Geometry: final body of the model. Coordinates: model frame, mm. A direction names the side the tool comes from. Give positions to 0.01 mm unless a question says otherwise; leave off trailing zeros. Order: outer loops, then holes, each group sorted by start corner. A loop starts at its lowest first (then second) coordinate and runs counter-clockwise, first axis right, second up. Notation, with made-up numbers: (87, 37) - (94, 37) arc R28 ccw to (94, 73) - close; hole circle Ø4 at (28.5, 21.5). An arc over 180 degrees is marked (long way). Use one line per item in the form item = value.
from build123d import *

# Parameters (mm, degrees)
SKETCH1_R             = 14.29385
SKETCH1_R_2           = 11.1125
BOSS_EXTRUDE1_DEPTH   = 6.35
CROQUIS1_R            = 2.38125
CORTAR_EXTRUIR1_DEPTH = 50
CROQUIS4_R            = 5
CORTAR_EXTRUIR2_DEPTH = 3.175
CROQUIS5_R            = 5
CORTAR_EXTRUIR3_DEPTH = 3.175
CROQUIS6_R            = 2.38125
CORTAR_EXTRUIR4_DEPTH = 10
CROQUIS7_R            = 2.38125
CORTAR_EXTRUIR5_DEPTH = 10
CROQUIS8_R            = 5
CORTAR_EXTRUIR6_DEPTH = 3.16


with BuildPart() as part:
    # Sketch1 → Boss-Extrude1 (new body)
    with BuildSketch(Plane.XY):
        with BuildLine():
            Line((0, 70), (310, 45))
            ThreePointArc((310, 45), (355, 0), (310, -45))
            Line((310, -45), (5.171398252, -69.808714643))
            ThreePointArc((5.171398252, -69.808714643), (-69.952162315, -2.587467389), (0, 70))
        make_face()
        Circle(SKETCH1_R, mode=Mode.SUBTRACT)
        with Locations((310, 0)):
            Circle(SKETCH1_R, mode=Mode.SUBTRACT)
        with Locations((162.878542763, 35)):
            Circle(SKETCH1_R_2, mode=Mode.SUBTRACT)
        with BuildLine():
            Line((107.898974887, 49.259511156), (143.314248041, 46.40344074))
            ThreePointArc((143.314248041, 46.40344074), (147.389908855, 43.644764005), (147.127454118, 38.730252238))
            Line((147.127454118, 38.730252238), (129.916226305, 11.754586611))
            ThreePointArc((129.916226305, 11.754586611), (125.651076231, 9.444205574), (121.433006579, 11.839462159))
            Line((121.433006579, 11.839462159), (103.228961238, 41.671198203))
            ThreePointArc((103.228961238, 41.671198203), (103.238833139, 46.896293531), (107.898974887, 49.259511156))
        make_face(mode=Mode.SUBTRACT)
        with BuildLine():
            Line((70.523244027, 6), (102.03004784, 6))
            ThreePointArc((102.03004784, 6), (106.3902351, 8.552804247), (106.298140539, 13.604493178))
            Line((106.298140539, 13.604493178), (96.590354482, 29.513051181))
            ThreePointArc((96.590354482, 29.513051181), (88.437172177, 34.296727565), (79.941746192, 30.151166228))
            Line((79.941746192, 30.151166228), (65.58297828, 10.229432452))
            ThreePointArc((65.58297828, 10.229432452), (67.271539685, 7.201787411), (70.523244027, 6))
        make_face(mode=Mode.SUBTRACT)
        with BuildLine():
            Line((219.623774494, 32.810522613), (206.130928429, 12.417497436))
            ThreePointArc((206.130928429, 12.417497436), (201.919524559, 10.176643248), (197.745901529, 12.48710226))
            Line((197.745901529, 12.48710226), (183.296864227, 35.133505128))
            ThreePointArc((183.296864227, 35.133505128), (183.227765467, 40.400743015), (187.913912204, 42.80669363))
            Line((187.913912204, 42.80669363), (215.855795571, 40.553315939))
            ThreePointArc((215.855795571, 40.553315939), (219.949772588, 37.757395035), (219.623774494, 32.810522613))
        make_face(mode=Mode.SUBTRACT)
        with BuildLine():
            Line((96.590354482, -29.513051181), (106.298140539, -13.604493178))
            ThreePointArc((106.298140539, -13.604493178), (106.3902351, -8.552804247), (102.03004784, -6))
            Line((102.03004784, -6), (70.523244027, -6))
            ThreePointArc((70.523244027, -6), (67.271539685, -7.201787411), (65.58297828, -10.229432452))
            Line((65.58297828, -10.229432452), (79.941746192, -30.151166228))
            ThreePointArc((79.941746192, -30.151166228), (88.437172177, -34.296727565), (96.590354482, -29.513051181))
        make_face(mode=Mode.SUBTRACT)
        with BuildLine():
            Line((187.913912204, -42.80669363), (215.855795571, -40.553315939))
            ThreePointArc((215.855795571, -40.553315939), (219.949772588, -37.757395035), (219.623774494, -32.810522613))
            Line((219.623774494, -32.810522613), (206.130928429, -12.417497436))
            ThreePointArc((206.130928429, -12.417497436), (201.919524559, -10.176643248), (197.745901529, -12.48710226))
            Line((197.745901529, -12.48710226), (183.296864227, -35.133505128))
            ThreePointArc((183.296864227, -35.133505128), (183.227765467, -40.400743015), (187.913912204, -42.80669363))
        make_face(mode=Mode.SUBTRACT)
        with BuildLine():
            Line((121.433006579, -11.839462159), (103.228961238, -41.671198203))
            ThreePointArc((103.228961238, -41.671198203), (103.238833139, -46.896293531), (107.898974887, -49.259511156))
            Line((107.898974887, -49.259511156), (143.314248041, -46.40344074))
            ThreePointArc((143.314248041, -46.40344074), (147.389908855, -43.644764005), (147.127454118, -38.730252238))
            Line((147.127454118, -38.730252238), (129.916226305, -11.754586611))
            ThreePointArc((129.916226305, -11.754586611), (125.651076231, -9.444205574), (121.433006579, -11.839462159))
        make_face(mode=Mode.SUBTRACT)
    extrude(amount=BOSS_EXTRUDE1_DEPTH)

    # Croquis1 → Cortar-Extruir1 (cut)
    with BuildSketch(Plane.XY.offset(6.35)):
        with Locations((98.995555235, -37.090103176)):
            Circle(CROQUIS1_R)
        with Locations((228.877351461, -26.519571404)):
            Circle(CROQUIS1_R)
    extrude(amount=-CORTAR_EXTRUIR1_DEPTH, mode=Mode.SUBTRACT)

    # Croquis4 → Cortar-Extruir2 (cut)
    with BuildSketch(Plane(origin=(0, 0, 0), x_dir=(-1, 0, 0), z_dir=(0, 0, -1))):
        with Locations((-228.877351461, -26.519571404)):
            Circle(CROQUIS4_R)
        with Locations((-98.995555235, -37.090103176)):
            Circle(CROQUIS4_R)
    extrude(amount=-CORTAR_EXTRUIR2_DEPTH, mode=Mode.SUBTRACT)

    # Croquis5 → Cortar-Extruir3 (cut)
    with BuildSketch(Plane(origin=(0, 0, 0), x_dir=(-1, 0, 0), z_dir=(0, 0, -1))):
        with Locations((-162.878542763, -5)):
            Circle(CROQUIS5_R)
    extrude(amount=-CORTAR_EXTRUIR3_DEPTH, mode=Mode.SUBTRACT)

    # Croquis6 → Cortar-Extruir4 (cut)
    with BuildSketch(Plane(origin=(0, 0, 0), x_dir=(-1, 0, 0), z_dir=(0, 0, -1))):
        with Locations((-162.878542763, -5)):
            Circle(CROQUIS6_R)
    extrude(amount=-CORTAR_EXTRUIR4_DEPTH, mode=Mode.SUBTRACT)

    # Croquis7 → Cortar-Extruir5 (cut)
    with BuildSketch(Plane(origin=(0, 0, 0), x_dir=(-1, 0, 0), z_dir=(0, 0, -1))):
        with Locations((-65.84135797, 50.868973694)):
            Circle(CROQUIS7_R)
        with Locations((-262.871569638, 39.210126075)):
            Circle(CROQUIS7_R)
    extrude(amount=-CORTAR_EXTRUIR5_DEPTH, mode=Mode.SUBTRACT)

    # Croquis8 → Cortar-Extruir6 (cut)
    with BuildSketch(Plane(origin=(0, 0, 0), x_dir=(-1, 0, 0), z_dir=(0, 0, -1))):
        with Locations((-262.871569638, 39.210126075)):
            Circle(CROQUIS8_R)
        with Locations((-65.84135797, 50.868973694)):
            Circle(CROQUIS8_R)
    extrude(amount=-CORTAR_EXTRUIR6_DEPTH, mode=Mode.SUBTRACT)


solid = part.part
(1) Ray query, line 1 along X through (y, z) = (-8, 6); line 2 along Y through (x, z) = (310, 2); line 3 along Y through (x, z) = (105, 6). Return the intervals inside material, ascending.
Computed values:
line_1 = -69.54 to -11.85, 11.85 to 66.52, 106.03 to 298.15, 321.85 to 354.28
line_2 = -45 to -14.29, 14.29 to 45
line_3 = -61.68 to -48.61, -38.77 to -15.73, -6.98 to 6.98, 15.73 to 38.77, 48.61 to 61.53
(2) Pull-direction query (X, two-part tool) for faces 1 (the face through (152.83, 57.675, 3.131)), 2 (the face through (145, 1, 0)), 3 (the face through (-1.861, 14.172, 3.131)); classes: released by +X, released by -X, zero draft, split by the parting line, or undercut.
Computed values:
face_1 = released by +X
face_2 = zero draft
face_3 = undercut
(3) Contact query for flat-ended pins moving along their axis: pin 1 Ø9 at (x, y) = (162.88, -5) entering from -Z (3 decimals); pin 2 Ø6 at (x, y) = (262.87, 39.21) entering from +Z; pin 3 Ø3 at (x, z) = (260, 3) entering from +Y; pin 4 Ø3 at (x, z) = (98.5, 4.5) entering from +Y. Output: stop coordinate, or through.
Computed values:
pin_1 = 3.175
pin_2 = 6.35
pin_3 = 49.15
pin_4 = 62.18
(4) Cut plane A-A on x = 302.5. Output: boundary loops of the cut face in (y, z), plus the area to 3 significant figures.
Computed values:
outline = (-45.61, 0) - (-12.17, 0) - (-12.17, 6.35) - (-45.61, 6.35) - close; (12.17, 0) - (45.6, 0) - (45.6, 6.35) - (12.17, 6.35) - close
area = 425 mm²
(5) Cut plane D-D on x = 21.5. Output: boundary loops of the cut face in (y, z), plus the area to 3 significant figures.
Computed values:
outline = (-68.48, 0) - (68.27, 0) - (68.27, 6.35) - (-68.48, 6.35) - close
area = 868 mm²
(6) Cut plane C-C on z = 1.25. Give the number of separate pieces and of enclosed holes in the cut face, plus the area to 3 significant figures.
Computed values:
separate_pieces = 1
enclosed_holes = 14
area = 39,200 mm²
(7) Cut plane B-B on x = 115. Output: boundary loops of the cut face in (y, z).
Computed values:
outline = (-60.87, 0) - (-48.69, 0) - (-48.69, 6.35) - (-60.87, 6.35) - close; (-22.38, 0) - (22.38, 0) - (22.38, 6.35) - (-22.38, 6.35) - close; (48.69, 0) - (60.73, 0) - (60.73, 6.35) - (48.69, 6.35) - close
(8) Reachability of faces 4 (the face through (72.66, -20.05, 3.13)), 5 (the face through (228, -29, 3.175)), 6 (the face through (145, 1, 6.35)) from +Z, -Z, +X, -X, +Y, -Y: full face, straight path, thin tool, end or side. Return the list, or none.
Computed values:
face_4 = +Z, -Z
face_5 = -Z
face_6 = +Z, +X, -X, +Y, -Y
